```python
from build123d import *

# Parameters (mm, degrees)
SKETCH1_W                = 33.02
SKETCH1_H                = 25.4
SKETCH1_R                = 1.4097
BOSS_EXTRUDE1_DEPTH      = 6.35
SKETCH2_W                = 33.02
SKETCH2_H                = 19.05
BOSS_EXTRUDE2_DEPTH      = 9.983600048
BOSS_EXTRUDE3_DEPTH      = 33.02
F_0_257_DIAMETER_HOLE1_D = 6.5278
CUT_EXTRUDE1_DEPTH       = 7.62
CHAMFER1_SIZE            = 1


with BuildPart() as part:
    # Sketch1 → Boss-Extrude1 (new body)
    with BuildSketch(Plane(origin=(0, 0, 0), x_dir=(0, 0, -1), z_dir=(1, 0, 0))):
        with Locations((16.51, -12.7)):
            Rectangle(SKETCH1_W, SKETCH1_H)
        with Locations((8.111016524, -7.0739)):
            Circle(SKETCH1_R, mode=Mode.SUBTRACT)
        with Locations((8.111016524, -18.3261)):
            Circle(SKETCH1_R, mode=Mode.SUBTRACT)
        with Locations((24.908983476, -18.3261)):
            Circle(SKETCH1_R, mode=Mode.SUBTRACT)
        with Locations((24.908983476, -7.0739)):
            Circle(SKETCH1_R, mode=Mode.SUBTRACT)
    extrude(amount=BOSS_EXTRUDE1_DEPTH)



with BuildPart() as body_2:
    # Sketch2 → Boss-Extrude2 (new body)
    with BuildSketch(Plane(origin=(6.35, 0, 0), x_dir=(0, 0, -1), z_dir=(1, 0, 0))):
        with Locations((16.51, 9.525)):
            Rectangle(SKETCH2_W, SKETCH2_H)
    extrude(amount=BOSS_EXTRUDE2_DEPTH)


with BuildPart() as part_1:
    add(part.part)

    add(body_2.part)  # Boss-Extrude3 merges body 2
    # Sketch3 → Boss-Extrude3 (add)
    with BuildSketch(Plane.XY):
        Polygon((6.35, 19.05), (0, 0), (6.35, 0), align=None)
    extrude(amount=-BOSS_EXTRUDE3_DEPTH)

    # F (0.257) Diameter Hole1 (through all)
    with Locations(Plane(origin=(16.333600048, 0, 0), x_dir=(0, 0, -1), z_dir=(1, 0, 0))):
        with Locations((7.62, 9.525), (25.4, 9.525)):
            Hole(F_0_257_DIAMETER_HOLE1_D / 2)

    # Sketch11 → Cut-Extrude1 (cut)
    with BuildSketch(Plane.ZY):
        with BuildLine():
            Line((-25.4, 15.113), (-7.62, 15.113))
            ThreePointArc((-7.62, 15.113), (-2.032, 9.525), (-7.62, 3.937))
            Line((-7.62, 3.937), (-25.4, 3.937))
            ThreePointArc((-25.4, 3.937), (-30.988, 9.525), (-25.4, 15.113))
        make_face()
    extrude(amount=-CUT_EXTRUDE1_DEPTH, mode=Mode.SUBTRACT)

    # Chamfer1
    chamfer1_edges = [part_1.edges().sort_by_distance(p)[0] for p in [
        (6.35, 0, -16.51),
    ]]
    chamfer(chamfer1_edges, length=CHAMFER1_SIZE)


solid = part_1.part
```
Build history of the part. All positions in model axes, mm. A direction names the side the tool comes from. Coordinates: 2 decimals unless noted, no trailing zeros. Write each loop counter-clockwise with the first axis right and the second up, starting at its lowest first coordinate (ties: lowest second). Pieces come first, ordered by that corner, then holes.
1. Band-saw the part on D-D, the plane y = -23. Give the cut face in (x, z).
Answer block:
outline: (0, -33.02) - (6.35, -33.02) - (6.35, 0) - (0, 0) - close
2. Band-saw the part on A-A, the plane y = -6.5. Give the cut face in (x, z), and give its area (3 significant figures).
Answer block:
outline: (0, -33.02) - (6.35, -33.02) - (6.35, -26.2) - (0, -26.2) - close; (0, -23.62) - (6.35, -23.62) - (6.35, -9.4) - (0, -9.4) - close; (0, -6.82) - (6.35, -6.82) - (6.35, 0) - (0, 0) - close
area: 177 mm2
3. Pull direction Y, two halves, no side cores. Call faces 1 (the flat face through (5.336, 16.008, -16.279)), 2 (the cylindrical face through (3.1, -18.3, -23.5)), 3 (the flat face through (6, 2, 0)): released by +Y, released by -Y, zero draft, split by the parting line, or undercut.
Answer block:
face 1: released by +Y
face 2: undercut
face 3: zero draft
4. Drop flat-ended pins along their axis: pin 1 (5 mm diameter, centred on x = 7.5, y = -16.5, fed in from +Z); pin 2 (5.5 mm diameter, centred on y = 7.5, z = -16, fed in from -X); pin 3 (2.5 mm diameter, centred on y = -18.33, z = -24.91, fed in from -X); pin 4 (3 mm diameter, centred on x = 13.5, z = -18, fed in from -Y). Give the stop position or say it passes through.
Answer block:
pin 1: stops at z = 0
pin 2: stops at x = 7.62
pin 3: passes through
pin 4: stops at y = 0
5. Band-saw the part on B-B, the plane z = -17.5. Give the cut face in (x, y), and give its area (3 significant figures).
Answer block:
outline: (0, -25.4) - (6.35, -25.4) - (6.35, -1) - (7.35, 0) - (16.33, 0) - (16.33, 19.05) - (6.35, 19.05) - (5.04, 15.11) - (7.62, 15.11) - (7.62, 3.94) - (1.31, 3.94) - (0, 0) - close
area: 363 mm2
6. 3-axis set-ups, long thin cutter, end or side, ignore diameter. For faces 4 (the cylindrical face through (11.92, 6.63, -6.11)), 5 (the cylindrical face through (5.12, 7.73, -2.33)): which of +Z, -Z, +X, -X, +Y, -Y reach the whole face in a straight line?
Answer block:
face 4: +X, -X
face 5: -X
7. Band-saw the part on C-C, the plane x = 10.25. Give the cut face in (y, z) (3 decimals), and give its area (3 significant figures).
Answer block:
outline: (0, -33.02) - (19.05, -33.02) - (19.05, 0) - (0, 0) - close; hole circle Ø6.528 at (9.525, -25.4); hole circle Ø6.528 at (9.525, -7.62)
area: 562 mm2
8. Drill centre lines: probe 1 along X at (y, z) = (6, -29.5); probe 2 along Y at (x, z) = (2.25, -20.5); probe 3 along X at (y, z) = (-6, -4). Where is each one in solid material? Low to high.
Answer block:
probe 1: x = 7.62 to 16.33
probe 2: y = -25.4 to 3.94
probe 3: x = 0 to 6.35
